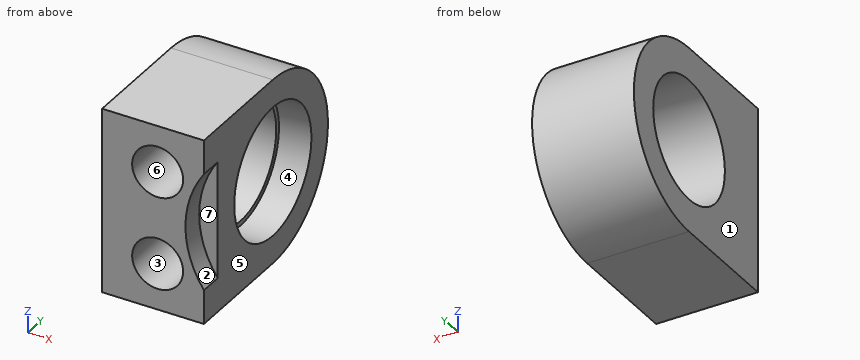
```python
from build123d import *

# Parameters (mm, degrees)
SKIZZE1_R                       = 6.5
AUFSATZ_LINEAR_AUSTRAGEN1_DEPTH = 11
SKIZZE2_R                       = 7
SCHNITT_LINEAR_AUSTRAGEN1_DEPTH = 3.5
SKIZZE3_R                       = 2.75
SCHNITT_LINEAR_AUSTRAGEN2_DEPTH = 6
SKIZZE4_R                       = 11
SCHNITT_LINEAR_AUSTRAGEN3_DEPTH = 2.5


with BuildPart() as part:
    # Skizze1 → Aufsatz-Linear austragen1 (new body)
    with BuildSketch(Plane(origin=(0, 0, 0), x_dir=(0, 0, -1), z_dir=(1, 0, 0))):
        with BuildLine():
            Line((-10, 0), (-10, -12.5))
            Line((-10, -12.5), (10, -12.5))
            Line((10, -12.5), (10, 0))
            ThreePointArc((10, 0), (0, 10), (-10, 0))
        make_face()
        Circle(SKIZZE1_R, mode=Mode.SUBTRACT)
    extrude(amount=AUFSATZ_LINEAR_AUSTRAGEN1_DEPTH)

    # Skizze2 → Schnitt-Linear austragen1 (cut)
    with BuildSketch(Plane(origin=(11, 0, 0), x_dir=(0, 0, -1), z_dir=(1, 0, 0))):
        Circle(SKIZZE2_R)
    extrude(amount=-SCHNITT_LINEAR_AUSTRAGEN1_DEPTH, mode=Mode.SUBTRACT)

    # Skizze3 → Schnitt-Linear austragen2 (cut)
    with BuildSketch(Plane.XZ.offset(12.5)):
        with Locations((6, 5)):
            Circle(SKIZZE3_R)
        with Locations((6, -5)):
            Circle(SKIZZE3_R)
    extrude(amount=-SCHNITT_LINEAR_AUSTRAGEN2_DEPTH, mode=Mode.SUBTRACT)

    # Skizze4 → Schnitt-Linear austragen3 (cut)
    with BuildSketch(Plane.XZ.offset(12.5)):
        with Locations((20, 0)):
            Circle(SKIZZE4_R)
    extrude(amount=-SCHNITT_LINEAR_AUSTRAGEN3_DEPTH, mode=Mode.SUBTRACT)


solid = part.part
```
The listing builds one solid part. Answer for the finished solid, in the listing's coordinates (mm). Face numbers are marked on the shaded views. A direction names the side the tool comes from. Coordinates: 2 decimals unless noted, no trailing zeros. Loops run counter-clockwise (first coordinate to the right, second up) from the corner with the lowest first, then second, coordinate; pieces in that order, holes last. Notation, with made-up numbers: (61.25, 21) -> (116.25, 21) arc R22 cw to (116.25, 59) -> close; hole circle Ø2 at (16.25, 25.5). An arc over 180 degrees is marked (long way). Return JSON: item names as keys, results as strings. Group by question number.
(1) A cutting plane is placed at B-B on x = 6. Write down the section's boundary in (y, z).
(2) Find the intervals of material crossed by probe 1 along Y at (x, z) = (2.5, 0); probe 2 along Y at (x, z) = (8.4, 0); probe 3 along Z at (x, y) = (2.75, -3.75), in increasing order. Write a range as from..to.
(3) A cutting plane is placed at A-A on z = 0. Write down the section's boundary in (x, y).
(4) A cutting plane is placed at D-D on z = 3.75. Write down the section's boundary in (x, y).
(5) Determine the mould class of the marked faces 1, 2, 3 and 4 for opening direction X: released by +X, released by -X, zero draft, split by the parting line, or undercut.
(6) A cutting plane is placed at C-C on y = 3.5. Write down the section's boundary in (x, z), and give its area (3 significant figures).
(7) Which of the six approach directions +Z, -Z, +X, -X, +Y, -Y give full straight-line access (tool end or side, diameter ignored) to the marked faces 5, 6 and 7?
(8) Given pin 1 Ø1.6 at (x, z) = (6, -4) entering from -Y; pin 2 Ø3 at (x, z) = (2, -4) entering from +Y; pin 3 Ø1.6 at (x, z) = (9.5, -3) entering from -Y, each flat-ended and moving along its own axis, determine where each tip first touches the part or whether it passes through.
The answers:
{
 "1": {"outline": "(-12.5, -10) -> (0, -10) arc R10 ccw to (0, 10) -> (-12.5, 10) -> (-12.5, 7.75) -> (-6.5, 7.75) -> (-6.5, 2.25) -> (-12.5, 2.25) -> (-12.5, -2.25) -> (-6.5, -2.25) -> (-6.5, -7.75) -> (-12.5, -7.75) -> close; hole circle Ø13 at (0, 0)"},
 "2": {"probe 1": "y = -12.5..-6.5, 6.5..10", "probe 2": "y = -12.5..-7, 7..10", "probe 3": "z = -10..-5.31, 5.31..10"},
 "3": {"outline": "(0, -12.5) -> (9, -12.5) -> (9, -10) -> (11, -10) -> (11, -7) -> (7.5, -7) -> (7.5, -6.5) -> (0, -6.5) -> close; (0, 6.5) -> (7.5, 6.5) -> (7.5, 7) -> (11, 7) -> (11, 10) -> (0, 10) -> close"},
 "4": {"outline": "(0, -12.5) -> (3.55, -12.5) -> (3.55, -6.5) -> (8.45, -6.5) -> (8.45, -12.5) -> (9.66, -12.5) -> (9.66, -10) -> (11, -10) -> (11, -5.91) -> (7.5, -5.91) -> (7.5, -5.31) -> (0, -5.31) -> close; (0, 5.31) -> (7.5, 5.31) -> (7.5, 5.91) -> (11, 5.91) -> (11, 9.27) -> (0, 9.27) -> close"},
 "5": {"face 1": "released by -X", "face 2": "released by +X", "face 3": "undercut", "face 4": "zero draft"},
 "6": {"outline": "(0, -9.37) -> (11, -9.37) -> (11, -6.06) -> (7.5, -6.06) -> (7.5, -5.48) -> (0, -5.48) -> close; (0, 5.48) -> (7.5, 5.48) -> (7.5, 6.06) -> (11, 6.06) -> (11, 9.37) -> (0, 9.37) -> close", "area": "81.5 mm^2"},
 "7": {"face 5": "+Z, -Z, +X, +Y, -Y", "face 6": "-Y", "face 7": "+X, -Y"},
 "8": {"pin 1": "stops at y = -6.5", "pin 2": "stops at y = 9.68", "pin 3": "stops at y = -12.5"}
}
